The listing builds one solid part. Answer for the finished solid, in the listing's coordinates (mm). Face numbers are marked on the shaded views. A direction names the side the tool comes from. Round coordinates to 2 decimals unless told otherwise and drop trailing zeros. Loops run counter-clockwise (first coordinate to the right, second up) from the corner with the lowest first, then second, coordinate; pieces in that order, holes last. Notation, with made-up numbers: (16.25, 43) -> (21.25, 43) arc R20 ccw to (21.25, 80) -> close; hole circle Ø4 at (-17.5, 35.5). An arc over 180 degrees is marked (long way). Use a Markdown table: item, result. Add a question column.
Q1. Section B-B on z = 8 is taken. Give the vertices of the cut face in (x, y), then the cut area to 3 significant figures.
Q2. Which of the six approach directions +Z, -Z, +X, -X, +Y, -Y give full straight-line access (tool end or side, diameter ignored) to the marked faces 1 and 2?
Q3. Section A-A on x = 0 is taken. Give the vertices of the cut face in (y, z), then the cut area to 3 significant figures.
Q4. Section C-C on y = -30.5 is taken. Give the vertices of the cut face in (x, z).
Q5. Given pin 1 Ø16 at (x, z) = (0, 38) entering from +Y; pin 2 Ø3 at (x, y) = (-50, 38) entering from +Z; pin 3 Ø1.5 at (y, z) = (1, 11.5) entering from +X; pin 4 Ø10 at (x, z) = (-102, 8) entering from +Y, each flat-ended and moving along its own axis, determine where each tip first touches the part or whether it passes through.
Q6. Consider line 1 (Z direction, x = 0, y = -1.5); line 2 (Z direction, x = 50.5, y = 26); line 3 (Y direction, x = 13.5, z = 42). Determine where each line is inside the solid, lowest interval first.
from build123d import *

# Parameters (mm, degrees)
F1_DEPTH = 2
F3_DEPTH = 2.5


with BuildPart() as f1:
    # F0 (on Top) → F1 (new body, symmetric)
    with BuildSketch(Plane.XY):
        with BuildLine():
            Line((49.1, 134.6), (-49.1, 134.6))
            ThreePointArc((-49.1, 134.6), (-109.5576297914, 109.5576297914), (-134.6, 49.1))
            Line((-134.6, 49.1), (-134.6, -49.1))
            ThreePointArc((-134.6, -49.1), (-109.5576297914, -109.5576297914), (-49.1, -134.6))
            Line((-49.1, -134.6), (49.1, -134.6))
            ThreePointArc((49.1, -134.6), (109.5576297914, -109.5576297914), (134.6, -49.1))
            Line((134.6, -49.1), (134.6, 49.1))
            ThreePointArc((134.6, 49.1), (109.5576297914, 109.5576297914), (49.1, 134.6))
        make_face()
    extrude(amount=F1_DEPTH, both=True)

    # F2 (on Front) → F3 (join, symmetric)
    with BuildSketch(Plane.XZ):
        with BuildLine():
            Line((-46.8736924231, 0), (0, 0))
            Line((0, 0), (46.8736924231, 0))
            Line((46.8736924231, 0), (46.8736924231, 18.0345661938))
            Line((46.8736924231, 18.0345661938), (11.3395565202, 50.4359355817))
            ThreePointArc((11.3395565202, 50.4359355817), (0, 54.829677236), (-11.3395565202, 50.4359355817))
            Line((-11.3395565202, 50.4359355817), (-46.8736924231, 18.0345661938))
            Line((-46.8736924231, 18.0345661938), (-46.8736924231, 0))
        make_face()
        with BuildLine():
            ThreePointArc((-3.666060556, 34.6), (-1.8261567868, 42.6545839116), (5, 38))
            ThreePointArc((5, 38), (4.6545839116, 36.1738432132), (3.666060556, 34.6))
            ThreePointArc((3.666060556, 34.6), (3.9156252517, 33.8172385748), (4, 33))
            ThreePointArc((4, 33), (3.7742546282, 31.6752351146), (3.1224989992, 30.5))
            ThreePointArc((3.1224989992, 30.5), (3.7742546282, 29.3247648854), (4, 28))
            ThreePointArc((4, 28), (-1.3247648854, 24.2257453718), (-3.1224989992, 30.5))
            ThreePointArc((-3.1224989992, 30.5), (-3.9653039239, 32.4742959088), (-3.666060556, 34.6))
        make_face(mode=Mode.SUBTRACT)
    extrude(amount=F3_DEPTH, both=True)


solid = f1.part
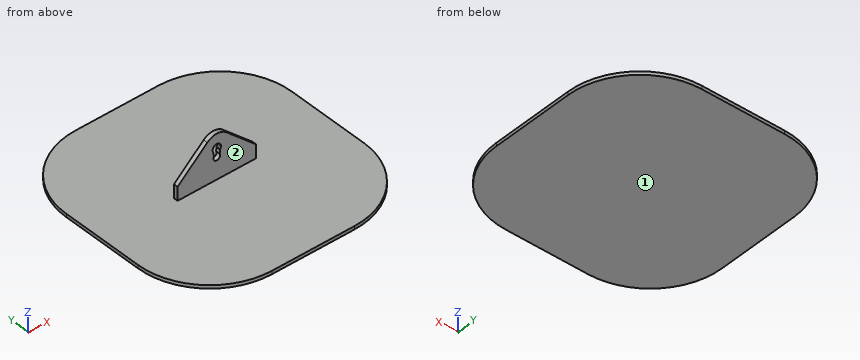
Checked values:
| question | item | result |
|---|---|---|
| 1 | outline | (-46.87, -2.5) -> (46.87, -2.5) -> (46.87, 2.5) -> (-46.87, 2.5) -> close |
| 1 | area | 469 mm2 |
| 2 | face 1 | -Z, +X, -X, +Y, -Y |
| 2 | face 2 | +Z, +X, -X, -Y |
| 3 | outline | (-134.6, -2) -> (134.6, -2) -> (134.6, 2) -> (2.5, 2) -> (2.5, 24) -> (-2.5, 24) -> (-2.5, 2) -> (-134.6, 2) -> close; (-2.5, 43) -> (2.5, 43) -> (2.5, 54.83) -> (-2.5, 54.83) -> close |
| 3 | area | 1,250 mm2 |
| 4 | outline | (-134.6, -2) -> (134.6, -2) -> (134.6, 2) -> (-134.6, 2) -> close |
| 5 | pin 1 | stops at y = 2.5 |
| 5 | pin 2 | stops at z = 2 |
| 5 | pin 3 | stops at x = 46.87 |
| 5 | pin 4 | passes through |
| 6 | line 1 | z = -2 to 24, 43 to 54.83 |
| 6 | line 2 | z = -2 to 2 |
| 6 | line 3 | y = -2.5 to 2.5 |
